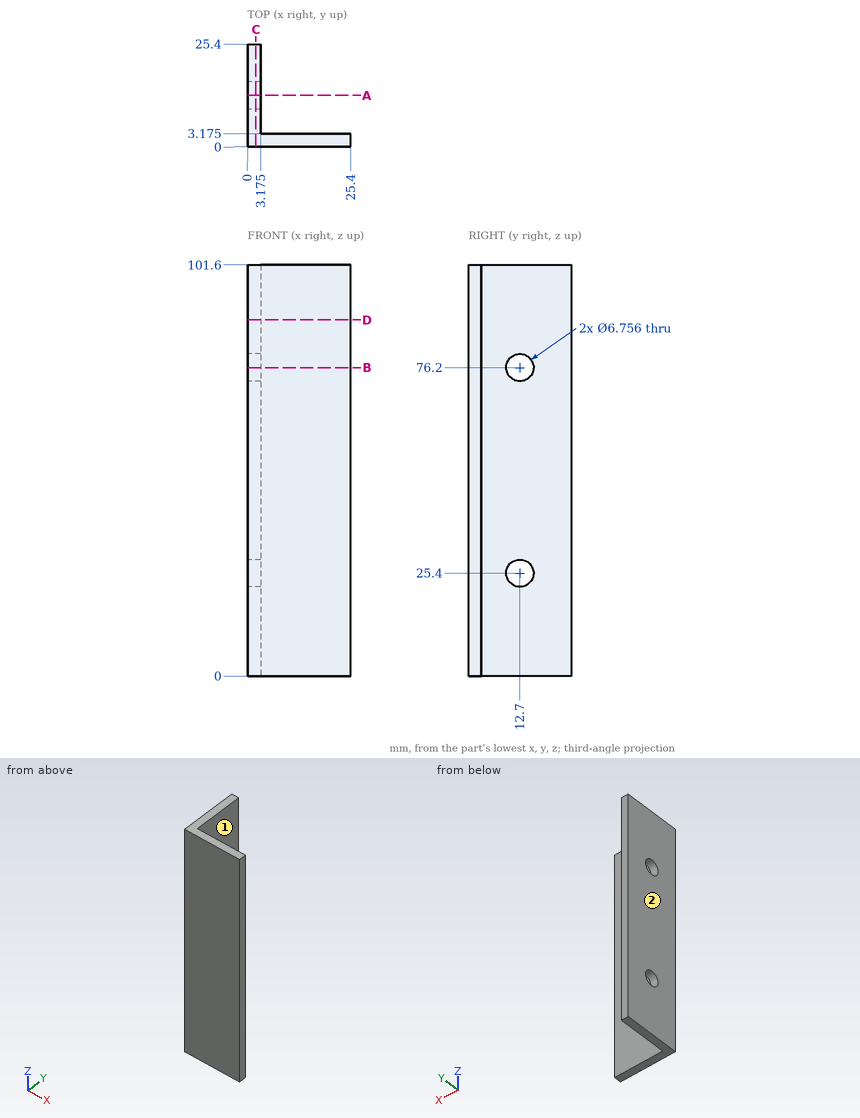
Source: three-view drawing plus pictorial views. Frame: mm from the lowest corner of the part. A direction names the side the tool comes from. Coordinates: 2 decimals unless noted, no trailing zeros. Order: outer loops, then holes, each group sorted by start corner. A loop starts at its lowest first (then second) coordinate and runs counter-clockwise, first axis right, second up.
1) Section D-D (z = 88). Return loops of the section in (x, y) (1 decimal), then the cut area to 3 significant figures.
Result sheet:
outline: (0, 0) - (25.4, 0) - (25.4, 3.2) - (3.2, 3.2) - (3.2, 25.4) - (0, 25.4) - close
area: 151 mm2
2) Section B-B (z = 76.2). Return loops of the section in (x, y) (1 decimal).
Result sheet:
outline: (0, 0) - (25.4, 0) - (25.4, 3.2) - (3.2, 3.2) - (3.2, 9.3) - (0, 9.3) - close; (0, 16.1) - (3.2, 16.1) - (3.2, 25.4) - (0, 25.4) - close
3) First-contact query: P1, Ø3, axis at y = 11.5, z = 44.5, coming from the +X side (3 decimals); P2, Ø10, axis at x = 19, z = 68.5, coming from the +Y side (3 decimals). Flat tips, straight axial feed; report the tip coordinate or a pass-through.
Result sheet:
P1: stops at x = 3.175
P2: stops at y = 3.175
4) Ray query, probe 1 along Z at (x, y) = (2.55, 12.7); probe 2 along Y at (x, z) = (0.75, 76.2); probe 3 along X at (y, z) = (19.5, 29) (1 decimal). Return the intervals inside material, ascending.
Result sheet:
probe 1: z = 0 to 22.02, 28.78 to 72.82, 79.58 to 101.6
probe 2: y = 0 to 9.32, 16.08 to 25.4
probe 3: x = 0 to 3.2
5) Set-up query: the marked faces 1 and 2. Return all of +Z, -Z, +X, -X, +Y, -Y with unobstructed straight access to the full face (end or side cutting, diameter ignored); none if empty.
Result sheet:
face 1: +Z, -Z, +X, +Y
face 2: +Z, -Z, -X, +Y, -Y
6) Section A-A (y = 12.7). Return loops of the section in (x, z) (1 decimal).
Result sheet:
outline: (0, 0) - (3.2, 0) - (3.2, 22) - (0, 22) - close; (0, 28.8) - (3.2, 28.8) - (3.2, 72.8) - (0, 72.8) - close; (0, 79.6) - (3.2, 79.6) - (3.2, 101.6) - (0, 101.6) - close
7) Section C-C (x = 2). Return loops of the section in (y, z).
Result sheet:
outline: (0, 0) - (25.4, 0) - (25.4, 101.6) - (0, 101.6) - close; hole circle Ø6.76 at (12.7, 25.4); hole circle Ø6.76 at (12.7, 76.2)
